```python
from build123d import *

# Parameters (mm, degrees)
SCHIZZO1_R                   = 42.562660939
ESTRUSIONE_ESTRUSIONE1_DEPTH = 5
SCHIZZO3_R                   = 11
TAGLIO_ESTRUSIONE2_DEPTH     = 6
SCHIZZO4_R                   = 1.5
SCHIZZO4_W                   = 5
SCHIZZO4_H                   = 30
SCHIZZO4_W_2                 = 30
SCHIZZO4_H_2                 = 5
TAGLIO_ESTRUSIONE3_DEPTH     = 6


with BuildPart() as part:
    # Schizzo1 → Estrusione-Estrusione1 (new body)
    with BuildSketch(Plane.XY):
        Circle(SCHIZZO1_R)
    extrude(amount=ESTRUSIONE_ESTRUSIONE1_DEPTH)

    # Schizzo3 → Taglio-Estrusione2 (cut, through all)
    with BuildSketch(Plane.XY):
        Circle(SCHIZZO3_R)
    extrude(amount=TAGLIO_ESTRUSIONE2_DEPTH, mode=Mode.SUBTRACT)

    # Schizzo4 → Taglio-Estrusione3 (cut, through all)
    with BuildSketch(Plane.XY):
        with Locations((17.67766953, 17.67766953)):
            Circle(SCHIZZO4_R)
        with Locations((17.67766953, -17.67766953)):
            Circle(SCHIZZO4_R)
        with Locations((-17.67766953, -17.67766953)):
            Circle(SCHIZZO4_R)
        with Locations((-17.67766953, 17.67766953)):
            Circle(SCHIZZO4_R)
        with Locations((-25, 0)):
            Rectangle(SCHIZZO4_W, SCHIZZO4_H)
        with Locations((0, 25)):
            Rectangle(SCHIZZO4_W_2, SCHIZZO4_H_2)
        with Locations((25, 0)):
            Rectangle(SCHIZZO4_W, SCHIZZO4_H)
        with Locations((0, -25)):
            Rectangle(SCHIZZO4_W_2, SCHIZZO4_H_2)
    extrude(amount=TAGLIO_ESTRUSIONE3_DEPTH, mode=Mode.SUBTRACT)


solid = part.part
```
Work out the finished part from the listing and answer in its coordinate system (mm). A direction names the side the tool comes from. Round coordinates to 2 decimals unless told otherwise and drop trailing zeros. Write each loop counter-clockwise with the first axis right and the second up, starting at its lowest first coordinate (ties: lowest second). Pieces come first, ordered by that corner, then holes.
1) Flat-ended cylindrical pins translate along their axes: P1, Ø1.5, axis at x = 5, z = 3.5, coming from the -Y side; P2, Ø1, axis at y = -29.5, z = 1.5, coming from the +X side; P3, Ø3, axis at x = 10, z = 0.5, coming from the -Y side. Find the tip coordinate at first contact, or state that the pin passes through.
2) A cutting plane is placed at C-C on x = 13. Determine the outline of the cut face in (y, z), and give its area (3 significant figures).
3) Which of the six approach directions +Z, -Z, +X, -X, +Y, -Y give full straight-line access (tool end or side, diameter ignored) to faces 1 (the face through (0, 27.5, 2)), 2 (the face through (9, -9, 0))?
4) A cutting plane is placed at B-B on x = -5.5. Determine the outline of the cut face in (y, z).
5) A cutting plane is placed at A-A on y = 0. Determine the outline of the cut face in (x, z).
6) Determine the mould class of faces 3 (the face through (-9.23, -41.55, 2.46)), 4 (the face through (9, -9, 5)), 5 (the face through (22.5, 0, 2)) for opening direction Y: pulls with the +Y half, pulls with the -Y half, needs draft (parallel to the pull), parting line crosses it, or undercut.
7) A cutting plane is placed at D-D on z = 2.35. Give the number of separate pieces and of enclosed holes in the cut face, and give its area (3 significant figures).
8) Consider probe 1 along X at (y, z) = (0.5, 4.4); probe 2 along Y at (x, z) = (0, 3.35); probe 3 along X at (y, z) = (1.5, 2.7). Determine where each line is inside the solid, lowest interval first.
Entries:
1. P1: stops at y = -42.35
1. P2: stops at x = 31.15
1. P3: stops at y = -41.71
2. outline: (-40.53, 0) - (-27.5, 0) - (-27.5, 5) - (-40.53, 5) - close; (-22.5, 0) - (22.5, 0) - (22.5, 5) - (-22.5, 5) - close; (27.5, 0) - (40.53, 0) - (40.53, 5) - (27.5, 5) - close
2. area: 355 mm2
3. face 1: +Z, -Z
3. face 2: -Z, +X, -X, +Y, -Y
4. outline: (-42.21, 0) - (-27.5, 0) - (-27.5, 5) - (-42.21, 5) - close; (-22.5, 0) - (-9.53, 0) - (-9.53, 5) - (-22.5, 5) - close; (9.53, 0) - (22.5, 0) - (22.5, 5) - (9.53, 5) - close; (27.5, 0) - (42.21, 0) - (42.21, 5) - (27.5, 5) - close
5. outline: (-42.56, 0) - (-27.5, 0) - (-27.5, 5) - (-42.56, 5) - close; (-22.5, 0) - (-11, 0) - (-11, 5) - (-22.5, 5) - close; (11, 0) - (22.5, 0) - (22.5, 5) - (11, 5) - close; (27.5, 0) - (42.56, 0) - (42.56, 5) - (27.5, 5) - close
6. face 3: parting line crosses it
6. face 4: needs draft
6. face 5: undercut
7. separate pieces: 1
7. enclosed holes: 9
7. area: 4,680 mm2
8. probe 1: x = -42.56 to -27.5, -22.5 to -10.99, 10.99 to 22.5, 27.5 to 42.56
8. probe 2: y = -42.56 to -27.5, -22.5 to -11, 11 to 22.5, 27.5 to 42.56
8. probe 3: x = -42.54 to -27.5, -22.5 to -10.9, 10.9 to 22.5, 27.5 to 42.54
